Could you check a few things on this drawing? It's one solid part, dimensions in mm from its lowest x, y, z. Give positions to 0.01 mm unless a question says otherwise; leave off trailing zeros. Loops run counter-clockwise (first coordinate to the right, second up) from the corner with the lowest first, then second, coordinate; pieces in that order, holes last.
Q1. I'm going to push flat-ended pins straight in: P1, Ø3, axis at y = 2, z = 32, coming from the -X side; P2, Ø3, axis at x = 24.5, y = 2.5, coming from the -Z side; P3, Ø1.9, axis at y = 2, z = 114.5, coming from the +X side. Where does each tip first touch, or does it pass through?
Q2. I need wall thicknesses on probe 1 along X at (y, z) = (2.75, 54.8); probe 2 along X at (y, z) = (3.25, 17) (1 decimal); probe 3 along Z at (x, y) = (41.5, 0.5). Which ranges of each line are inside material? Lowest first, please.
Q3. Suppose I cut it at C-C (y = 5.25). Count the separate pieces of the cut face and the enclosed holes in it, and give its area (3 significant figures).
Q4. Suppose I cut it at B-B (x = 58). List the corners of the cut face in (y, z) for me.
Q5. Suppose I cut it at A-A (z = 54.8). List the corners of the cut face in (x, y) for me.
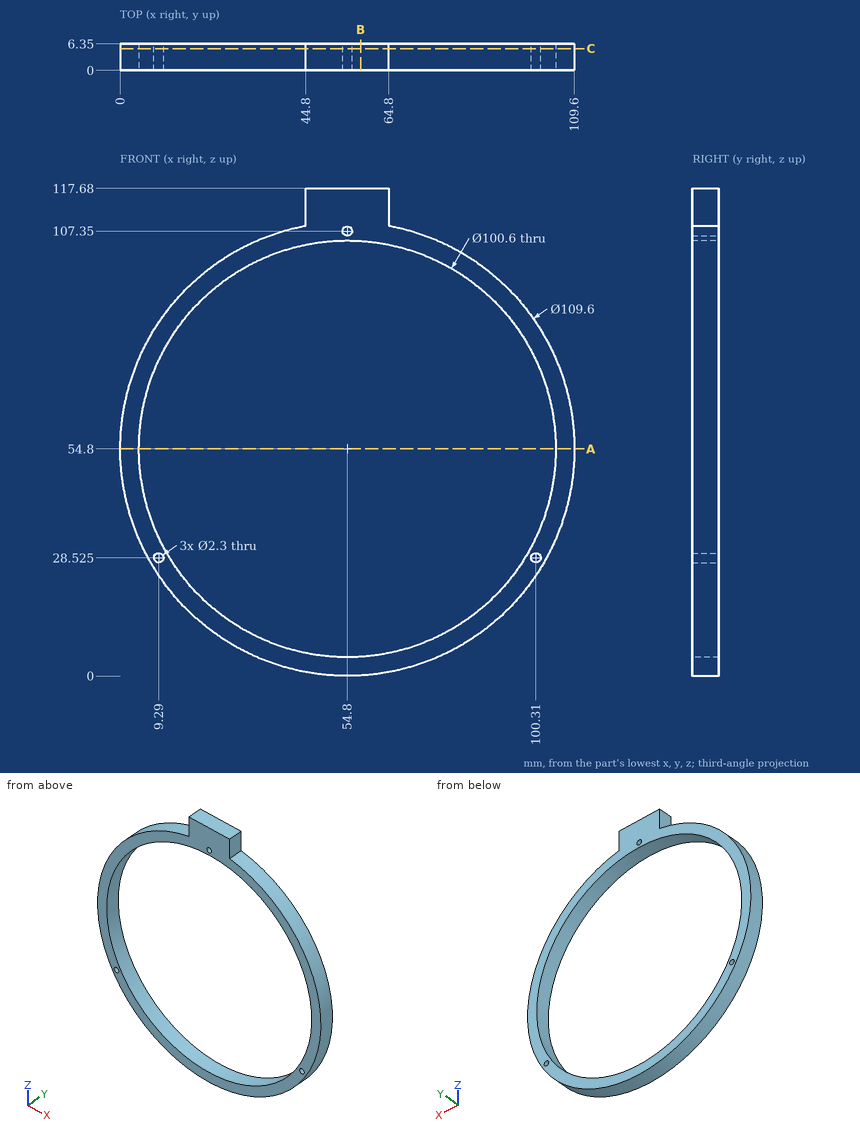
Solutions:
1. P1: stops at x = 4.31
1. P2: stops at z = 8.18
1. P3: stops at x = 64.8
2. probe 1: x = 0 to 4.5, 105.1 to 109.6
2. probe 2: x = 15.1 to 21.6, 88 to 94.5
2. probe 3: z = 1.64 to 6.29, 103.31 to 107.96
3. separate pieces: 1
3. enclosed holes: 4
3. area: 1,640 mm2
4. outline: (0, 0.09) - (6.35, 0.09) - (6.35, 4.6) - (0, 4.6) - close; (0, 105) - (6.35, 105) - (6.35, 117.68) - (0, 117.68) - close
5. outline: (0, 0) - (4.5, 0) - (4.5, 6.35) - (0, 6.35) - close; (105.1, 0) - (109.6, 0) - (109.6, 6.35) - (105.1, 6.35) - close
